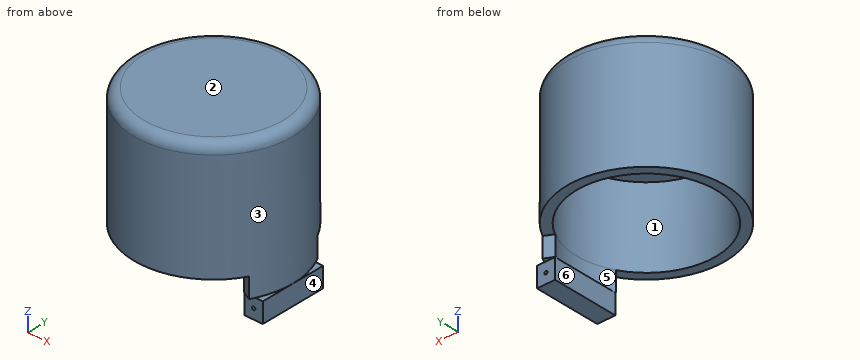
Autodesk Inventor part; units mm, degrees
ref_plane "YZ Plane" through (0, 0, 0) normal (1, 0, 0) x (0, 1, 0)
ref_plane "XZ Plane" through (0, 0, 0) normal (0, 1, 0) x (-1, 0, 0)
ref_plane "XY Plane" through (0, 0, 0) normal (0, 0, 1) x (1, 0, 0)
sketch "Sketch1" plane through (0, 0, 0) normal (0, 0, 1) x (1, 0, 0)
  circle A0 centre (-4.4309, 2.4544) radius 22.335
  circle A1 centre (-4.4309, 2.4544) radius 25.4
  point P0 (0, 0)
  dimension "d0" = 44.67
  dimension "d1" = 50.8
extrude "Extrusion1" add sketch "Sketch1" along normal blind 25.4
sketch "Sketch2" plane through (-4.4309, 2.4544, 25.4) normal (0, 0, 1) x (1, 0, 0)
  circle A0 centre (0, 0) radius 25.4
  point P0 (4.4309, -2.4544)
extrude "Extrusion2" add sketch "Sketch2" along normal blind 12.7
fillet "Fillet1" radius 3.175 1 edges at (-29.8309, 2.4544, 38.1)
sketch "Sketch3" plane through (-4.4309, 2.4544, 0) normal (0, 0, -1) x (-1, 0, 0)
  circle A0 centre (0, 0) radius 25.4
  arc A1 (-22.2614, 12.2307) -> (-22.2614, -12.2307) centre (0, 0) ccw
  line L0 (-22.2614, 12.2307) -> (-22.2614, -12.2307) construction
  line L1 (-22.2614, 12.2307) -> (2.1999, 12.2307) construction
  circle A2 centre (0, 0) radius 22.225
  arc A3 (-19.4415, 10.7694) -> (-19.4415, -10.7694) centre (0, 0) ccw
  line L2 (-19.4415, 10.7694) -> (-19.4415, -10.7694) construction
  line L3 (-19.4415, 10.7694) -> (2.0972, 10.7694) construction
  line L4 (-22.2614, -12.2307) -> (-19.4415, -10.7694)
  line L5 (-22.2614, 12.2307) -> (-19.4415, 10.7694)
  point P0 (-4.4309, -2.4544)
  dimension "d7" = 90
  dimension "d8" = 90
extrude "Extrusion3" add sketch "Sketch3" along normal blind 6.35 contours L5 A2 L4 A0 picked at (-24.2184, -0.7482)
sketch "Sketch4" plane through (-4.4309, 2.4544, -6.35) normal (0, 0, -1) x (-1, 0, 0)
  circle A0 centre (0, 0) radius 22.335
  line L0 (-19.5898, 10.728) -> (-25.4, 10.728)
  line L1 (-25.4, 10.728) -> (-25.4, -10.7831)
  line L2 (-25.4, -10.7831) -> (-19.5898, -10.7831)
  line L3 (-19.5898, -10.7831) -> (-19.5898, 10.728)
  point P0 (-4.4309, -2.4544)
extrude "Extrusion4" add sketch "Sketch4" along normal blind 6.35 contours L3 A0 | A0 L3 L2 L1 L0 picked at (-20.171, -2.2046)
sketch "Sketch5" plane through (-4.4309, 2.4544, -6.35) normal (0, 0, -1) x (-1, 0, 0)
  point P0 (-4.4309, -2.4544)
sketch "Sketch6" plane through (18.5665, -8.3288, -6.35) normal (0, -1, 0) x (1, 0, 0)
  line L0 (-3.4076, -6.35) -> (2.4025, -6.35)
  line L1 (-3.4076, 0) -> (0, 0)
  line L2 (2.4025, -6.35) -> (-3.4076, 0) construction
  line L3 (-3.4076, -6.35) -> (2.4025, 0) construction
  line L4 (2.4025, 0) -> (2.4025, 41.275)
  circle A0 centre (-0.5026, -3.175) radius 0.5
  point P0 (-18.5665, 6.35)
  dimension "d13" = 1
extrude "Extrusion5" cut sketch "Sketch6" against normal blind 25.4
properties part number "ballcarriage"
Input: part model. Units: mm. Frame: model coordinates. Face numbers are marked on the shaded views. A direction names the side the tool comes from. Coordinates: 2 decimals unless noted, no trailing zeros. Loops run counter-clockwise (first coordinate to the right, second up) from the corner with the lowest first, then second, coordinate; pieces in that order, holes last.
Q1. Material intervals for line 1 (X direction, y = 0.5, z = -9.5); line 2 (Y direction, x = -4, z = 11); line 3 (Y direction, x = -12.5, z = 10), sorted ascending.
Q2. Draft query along Y for the marked faces 1, 2 and 3. Return one class per face: +Y half, -Y half, draft (parallel to the pull), parting line (faces both ways), or undercut.
Q3. Cut plane A-A (z = 5.5). Output: boundary loops of the cut face in (x, y) (3 decimals).
Q4. Contact query for flat-ended pins moving along their axis: pin 1 (3 mm diameter, centred on x = 7.5, z = 4.5, fed in from +Y); pin 2 (4.5 mm diameter, centred on x = 17.5, z = -10.5, fed in from +Y); pin 3 (6 mm diameter, centred on x = -11.5, y = 2.5, fed in from -Z). Output: stop coordinate, or through.
Q5. Set-up query: the marked faces 4, 5 and 6. Return all of +Z, -Z, +X, -X, +Y, -Y with unobstructed straight access to the full face (end or side cutting, diameter ignored); none if empty.
Working result:
1. line 1: x = 15.16 to 17.56, 18.56 to 20.97
1. line 2: y = -22.94 to -19.88, 24.79 to 27.85
1. line 3: y = -21.63 to -18.37, 23.28 to 26.54
2. face 1: undercut
2. face 2: draft
2. face 3: parting line
3. outline: circle Ø50.8 at (-4.431, 2.454); hole circle Ø44.67 at (-4.431, 2.454)
4. pin 1: stops at y = 25.61
4. pin 2: stops at y = 13.18
4. pin 3: stops at z = 25.4
5. face 4: +Z, -Z, +X, +Y, -Y
5. face 5: -X
5. face 6: -Z, -X, +Y, -Y
